For this review, take the finished solid that the model builds, in its own axes (mm). Coordinates: 2 decimals unless noted, no trailing zeros. Loops run counter-clockwise (first coordinate to the right, second up) from the corner with the lowest first, then second, coordinate; pieces in that order, holes last. Notation, with made-up numbers: M 45,27 L 102,27 A20 cw 102,43 Z; hole C 82.5,37.25 d8. An arc over 180 degrees is marked long. Answer as a JSON object with one key per item and string values. Group by question number.
Item 1: Wall thickness on L1, parallel to X at y = 47, z = 297.5; L2, parallel to X at y = 20.5, z = 251; L3, parallel to Z at x = -1334, y = 20: over which ranges is each line inside the solid? List them lowest first. Write a range as from..to.
Item 2: Add section A-A (x = -332.5). State the section outline as (y, z) points.
Item 3: Add section B-B (z = 768). State the section outline as (x, y) points.
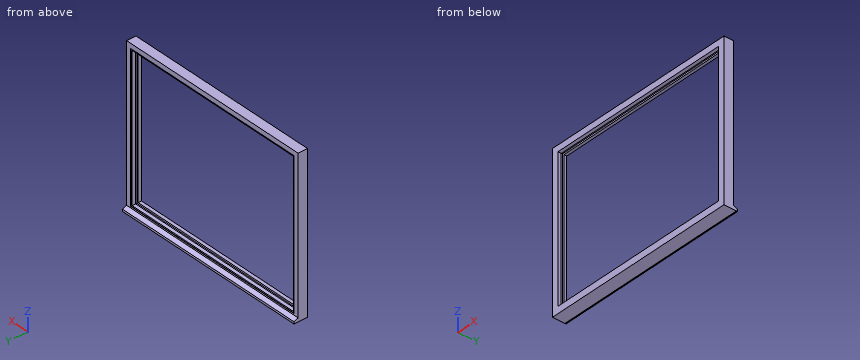
from build123d import *

# Parameters (mm, degrees)
F1_DEPTH = 1890
F3_DEPTH = 1490


with BuildPart() as f1:
    # F0 (on Right) → F1 (new body)
    with BuildSketch(Plane.YZ):
        with BuildLine():
            Line((0, 40), (0, 0))
            Line((0, 0), (119, 0))
            ThreePointArc((119, 0), (122, 3), (125, 0))
            Line((125, 0), (130, 0))
            Line((130, 0), (130, 20))
            Line((130, 20), (90, 35.704561))
            Line((90, 35.704561), (90, 50))
            Line((90, 50), (87, 50))
            Line((87, 50), (57, 50))
            Line((57, 50), (32, 50))
            Line((32, 50), (32, 65))
            Line((32, 65), (0, 65))
            Line((0, 65), (0, 40))
        make_face()
        Polygon((57, 65), (57, 50), (87, 50), (87, 62), align=None)
        Polygon((87, 1433), (87, 1445), (57, 1445), (57, 1430), align=None)
        Polygon((90, 1490), (0, 1490), (0, 1430), (32, 1430), (32, 1445), (57, 1445), (87, 1445), (90, 1445), align=None)
    extrude(amount=-F1_DEPTH)

    # F2 (on face) → F3 (join)
    with BuildSketch(Plane.XY.offset(1490)):
        Polygon((-60, 0), (0, 0), (0, 90), (-45, 90), (-45, 87), (-45, 57), (-45, 32), (-60, 32), align=None)
        Polygon((-45, 57), (-45, 87), (-57, 87), (-60, 57), align=None)
        Polygon((-1890, 90), (-1890, 0), (-1830, 0), (-1830, 32), (-1845, 32), (-1845, 57), (-1845, 87), (-1845, 90), align=None)
        Polygon((-1833, 87), (-1845, 87), (-1845, 57), (-1830, 57), align=None)
    extrude(amount=-F3_DEPTH)


solid = f1.part
From the geometry:
{
 "1": {"L1": "x = -1890..-1845, -45..0", "L2": "x = -1890..-1830, -60..0", "L3": "z = 0..65, 1430..1490"},
 "2": {"outline": "M 0,0 L 119,0 A3 cw 125,0 L 130,0 L 130,20 L 90,35.7 L 90,50 L 87,50 L 87,62 L 57,65 L 57,50 L 32,50 L 32,65 L 0,65 Z; M 0,1430 L 32,1430 L 32,1445 L 57,1445 L 57,1430 L 87,1433 L 87,1445 L 90,1445 L 90,1490 L 0,1490 Z"},
 "3": {"outline": "M -1890,0 L -1830,0 L -1830,32 L -1845,32 L -1845,57 L -1830,57 L -1833,87 L -1845,87 L -1845,90 L -1890,90 Z; M -60,0 L 0,0 L 0,90 L -45,90 L -45,87 L -57,87 L -60,57 L -45,57 L -45,32 L -60,32 Z"}
}
